Check sheet for the modelled part. Datum: model origin and axes. Units: mm. A direction names the side the tool comes from. Round coordinates to 2 decimals unless told otherwise and drop trailing zeros. Order: outer loops, then holes, each group sorted by start corner. A loop starts at its lowest first (then second) coordinate and runs counter-clockwise, first axis right, second up.
(1) Depth check by flat-ended pin: pin 1 (6 mm diameter, centred on y = 3, z = 22, fed in from -X); pin 2 (9 mm diameter, centred on y = -1, z = 22, fed in from +X); pin 3 (2 mm diameter, centred on y = 3, z = 30, fed in from +X); pin 4 (10 mm diameter, centred on x = -55.5, z = -14.5, fed in from +Y). Enter the tip coordinate at first touch or a pass-through.
(2) Sectioned sample at D-D, the plane x = 16.5. Enter the section's corners in (y, z), and give its area (3 significant figures).
(3) Sectioned sample at C-C, the plane x = 42.5. Enter the section's corners in (y, z).
(4) Tool access check on faces 5 (the flat face through (0, 9.5, 7)), 6 (the flat face through (12.5, 0, -19)), 7 (the cylindrical face through (-14.985, 7.944, -0.66)). Record the directions out of +Z, -Z, +X, -X, +Y, -Y that give a thin tool (end or side, any length) a straight path to the whole face; none if there is none.
(5) Thickness scan on probe 1 along X at (y, z) = (1.25, 0); probe 2 along Z at (x, y) = (0, 3.5); probe 3 along X at (y, z) = (4.5, 0). Record the ranges inside material, lowest first.
(6) Sectioned sample at B-B, the plane z = 0. Enter the section's corners in (x, y), and give its area (3 significant figures).
(7) Mould release check, pull along X, two halves, no side actions. Record for faces 1 (the flat face through (-37.15, 0.056, -10.035)), 2 (the cylindrical face through (37.505, 0.056, -0.22)), 3 (the cylindrical face through (-6, 11, 0)), 4 (the flat face through (12.5, 0, 19)): released by +X, released by -X, zero draft, split by the parting line, or undercut.
(8) Sectioned sample at A-A, the plane x = 0. Enter the section's corners in (y, z), and give its area (3 significant figures).
```python
from build123d import *

# Parameters (mm, degrees)
SKETCH1_R           = 10
BOSS_EXTRUDE1_DEPTH = 4
SKETCH2_R           = 15
SKETCH2_R_2         = 10
BOSS_EXTRUDE2_DEPTH = 8
SKETCH3_R           = 5
CUT_EXTRUDE1_DEPTH  = 9
BOSS_EXTRUDE3_START = 9.5
SKETCH4_R           = 10
SKETCH4_R_2         = 6
BOSS_EXTRUDE3_DEPTH = 2.5


with BuildPart() as part:
    # Sketch1 → Boss-Extrude1 (new body, symmetric)
    with BuildSketch(Plane(origin=(0, 0, 0), x_dir=(1, 0, 0), z_dir=(0, 1, 0))):
        with BuildLine():
            Line((12.5, 12.5), (12.5, 26.25))
            ThreePointArc((12.5, 26.25), (0, 38.75), (-12.5, 26.25))
            Line((-12.5, 26.25), (-12.5, 12.5))
            Line((-12.5, 12.5), (-62.5, 7.5))
            ThreePointArc((-62.5, 7.5), (-70, 0), (-62.5, -7.5))
            Line((-62.5, -7.5), (-12.5, -12.5))
            Line((-12.5, -12.5), (-12.5, -26.25))
            ThreePointArc((-12.5, -26.25), (0, -38.75), (12.5, -26.25))
            Line((12.5, -26.25), (12.5, -12.5))
            Line((12.5, -12.5), (62.5, -7.5))
            ThreePointArc((62.5, -7.5), (70, 0), (62.5, 7.5))
            Line((62.5, 7.5), (12.5, 12.5))
        make_face()
        Circle(SKETCH1_R, mode=Mode.SUBTRACT)
    extrude(amount=BOSS_EXTRUDE1_DEPTH, both=True)

    # Sketch2 → Boss-Extrude2 (add)
    with BuildSketch(Plane(origin=(0, 4, 0), x_dir=(1, 0, 0), z_dir=(0, 1, 0))):
        Circle(SKETCH2_R)
        Circle(SKETCH2_R_2, mode=Mode.SUBTRACT)
    extrude(amount=BOSS_EXTRUDE2_DEPTH)

    # Sketch3 → Cut-Extrude1 (cut, through all)
    with BuildSketch(Plane(origin=(0, 4, 0), x_dir=(1, 0, 0), z_dir=(0, 1, 0))):
        with Locations((42.5, 0)):
            Circle(SKETCH3_R)
        with Locations((-42.5, 0)):
            Circle(SKETCH3_R)
    extrude(amount=-CUT_EXTRUDE1_DEPTH, mode=Mode.SUBTRACT)

    # Sketch4 → Boss-Extrude3 (add)
    with BuildSketch(Plane(origin=(0, 0, 0), x_dir=(1, 0, 0), z_dir=(0, 1, 0)).offset(BOSS_EXTRUDE3_START)):
        Circle(SKETCH4_R)
        Circle(SKETCH4_R_2, mode=Mode.SUBTRACT)
    extrude(amount=BOSS_EXTRUDE3_DEPTH)


solid = part.part
```
Derived:
1. pin 1: stops at x = -12.5
1. pin 2: stops at x = 12.5
1. pin 3: stops at x = 12.19
1. pin 4: passes through
2. outline: (-4, -12.1) - (4, -12.1) - (4, 12.1) - (-4, 12.1) - close
2. area: 194 mm2
3. outline: (-4, -9.5) - (4, -9.5) - (4, -5) - (-4, -5) - close; (-4, 5) - (4, 5) - (4, 9.5) - (-4, 9.5) - close
4. face 5: -Y
4. face 6: -Z, +X, +Y, -Y
4. face 7: +Y
5. probe 1: x = -70 to -47.5, -37.5 to -10, 10 to 37.5, 47.5 to 70
5. probe 2: z = -38.75 to -10, 10 to 38.75
5. probe 3: x = -15 to -10, 10 to 15
6. outline: (-70, -4) - (-47.5, -4) - (-47.5, 4) - (-70, 4) - close; (-37.5, -4) - (-10, -4) - (-10, 9.5) - (-6, 9.5) - (-6, 12) - (-15, 12) - (-15, 4) - (-37.5, 4) - close; (6, 9.5) - (10, 9.5) - (10, -4) - (37.5, -4) - (37.5, 4) - (15, 4) - (15, 12) - (6, 12) - close; (47.5, -4) - (70, -4) - (70, 4) - (47.5, 4) - close
6. area: 900 mm2
7. face 1: released by -X
7. face 2: undercut
7. face 3: undercut
7. face 4: released by +X
8. outline: (-4, -38.75) - (4, -38.75) - (4, -15) - (12, -15) - (12, -6) - (9.5, -6) - (9.5, -10) - (-4, -10) - close; (-4, 10) - (9.5, 10) - (9.5, 6) - (12, 6) - (12, 15) - (4, 15) - (4, 38.75) - (-4, 38.75) - close
8. area: 560 mm2
